```python
from build123d import *

# Parameters (mm, degrees)
F1_DEPTH = 10.16


with BuildPart() as f1:
    # F0 (on Front) → F1 (new body, symmetric)
    with BuildSketch(Plane.XZ):
        Polygon((158.686374, 147.795809), (-146.113626, 147.795809), (-146.113626, -157.004191), (-90.020779, -157.004191), (-90.020779, -92.344157), (-51.920779, -92.344157), (-51.920779, -157.004191), (-13.820779, -157.004191), (-13.820779, -92.344157), (24.279221, -92.344157), (24.279221, -157.004191), (62.379221, -157.004191), (62.379221, -92.344157), (100.479221, -92.344157), (100.479221, -157.004191), (158.686374, -157.004191), align=None)
    extrude(amount=F1_DEPTH, both=True)


solid = f1.part
```
Part model, mm, in its own coordinate system. A direction names the side the tool comes from. Round coordinates to 2 decimals unless told otherwise and drop trailing zeros. Loops run counter-clockwise (first coordinate to the right, second up) from the corner with the lowest first, then second, coordinate; pieces in that order, holes last.
1. Two-plate mould, pull along X, no slides. Class faces 1 (the face through (-90.021, 0, -125)), 2 (the face through (4, 10.16, -2)), 3 (the face through (-146.114, 0, -2)): pulls with the +X half, pulls with the -X half, needs draft (parallel to the pull), parting line crosses it, or undercut.
Solutions:
face 1: undercut
face 2: needs draft
face 3: pulls with the -X half
2. 3-axis set-ups, long thin cutter, end or side, ignore diameter. For faces 4 (the face through (-33, 0, -157.004)), 5 (the face through (81, 0, -92.344)): which of +Z, -Z, +X, -X, +Y, -Y reach the whole face in a straight line?
Solutions:
face 4: -Z, +X, -X, +Y, -Y
face 5: -Z, +Y, -Y
3. Slice it at C-C (x = -68.5). Give the cut face in (y, z), and give its area (3 significant figures).
Solutions:
outline: (-10.16, -92.34) - (10.16, -92.34) - (10.16, 147.8) - (-10.16, 147.8) - close
area: 4,880 mm2
4. Slice it at B-B (y = 6.25). Give the cut face in (x, z).
Solutions:
outline: (-146.11, -157) - (-90.02, -157) - (-90.02, -92.34) - (-51.92, -92.34) - (-51.92, -157) - (-13.82, -157) - (-13.82, -92.34) - (24.28, -92.34) - (24.28, -157) - (62.38, -157) - (62.38, -92.34) - (100.48, -92.34) - (100.48, -157) - (158.69, -157) - (158.69, 147.8) - (-146.11, 147.8) - close
5. Flat gauge pin, fed straight in: pin 1 (10 mm diameter, centred on x = 8, y = 2, fed in from -Z). Where does the tip first touch, or does it go through?
Solutions:
pin 1: stops at z = -92.34
6. Drill centre lines: line 1 along X through (y, z) = (-5.5, -104); line 2 along Z through (x, y) = (-72, 0). Where is each one in solid material? Low to high.
Solutions:
line 1: x = -146.11 to -90.02, -51.92 to -13.82, 24.28 to 62.38, 100.48 to 158.69
line 2: z = -92.34 to 147.8
7. Slice it at A-A (z = -98). Give the cut face in (x, y), and give its area (3 significant figures).
Solutions:
outline: (-146.11, -10.16) - (-90.02, -10.16) - (-90.02, 10.16) - (-146.11, 10.16) - close; (-51.92, -10.16) - (-13.82, -10.16) - (-13.82, 10.16) - (-51.92, 10.16) - close; (24.28, -10.16) - (62.38, -10.16) - (62.38, 10.16) - (24.28, 10.16) - close; (100.48, -10.16) - (158.69, -10.16) - (158.69, 10.16) - (100.48, 10.16) - close
area: 3,870 mm2
